```python
from build123d import *

# Parameters (mm, degrees)
CROQUIS1_W              = 30
CROQUIS1_H              = 30
SALIENTE_EXTRUIR1_DEPTH = 200
CROQUIS2_R              = 2
CORTAR_EXTRUIR1_DEPTH   = 25
CROQUIS3_R              = 2
CORTAR_EXTRUIR2_DEPTH   = 203.792997907
CROQUIS4_R              = 2
CORTAR_EXTRUIR3_DEPTH   = 25


with BuildPart() as part:
    # Croquis1 → Saliente-Extruir1 (new body)
    with BuildSketch(Plane.XY):
        Rectangle(CROQUIS1_W, CROQUIS1_H)
    extrude(amount=SALIENTE_EXTRUIR1_DEPTH)

    # Croquis2 → Cortar-Extruir1 (cut)
    with BuildSketch(Plane.XY.offset(200)):
        with Locations((-7.221825407, 7.221825407)):
            Circle(CROQUIS2_R)
        with Locations(Location((7.221825407, -7.221825407, 0), (0, 0, 180))):
            Circle(CROQUIS2_R)
    extrude(amount=-CORTAR_EXTRUIR1_DEPTH, mode=Mode.SUBTRACT)

    # Croquis3 → Cortar-Extruir2 (cut, through all)
    with BuildSketch(Plane(origin=(0, 15, 0), x_dir=(1, 0, 0), z_dir=(0, 1, 0))):
        with Locations(Location((0, -196, 0), (0, 0, 270))):
            Circle(CROQUIS3_R)
    extrude(amount=-CORTAR_EXTRUIR2_DEPTH, mode=Mode.SUBTRACT)

    # Croquis4 → Cortar-Extruir3 (cut)
    with BuildSketch(Plane(origin=(0, 0, 0), x_dir=(-1, 0, 0), z_dir=(0, 0, -1))):
        Circle(CROQUIS4_R)
    extrude(amount=-CORTAR_EXTRUIR3_DEPTH, mode=Mode.SUBTRACT)


solid = part.part
```
Input: part model. Units: mm. Frame: model coordinates. A direction names the side the tool comes from. Coordinates: 2 decimals unless noted, no trailing zeros. Loops run counter-clockwise (first coordinate to the right, second up) from the corner with the lowest first, then second, coordinate; pieces in that order, holes last. Notation, with made-up numbers: (-12, 71.25) -> (11, 71.25) arc R17 ccw to (11, 95.25) -> close; hole circle Ø10 at (85, -12.75). An arc over 180 degrees is marked (long way). Use a Markdown table: item, result.
1) Access query for faces 4 (the cylindrical face through (9.22, -7.31, 187.68)), 5 (the cylindrical face through (0, -2, 12)), 6 (the cylindrical face through (0, 0, 194)). Directions: +Z, -Z, +X, -X, +Y, -Y. A direction counts if a zero-diameter tool reaches every point of the face in a straight line with its end or side. Return the directions, or none.
Results found:
| item | result |
|---|---|
| face 4 | +Z |
| face 5 | -Z |
| face 6 | +Y, -Y |
2) Contact query for flat-ended pins moving along their axis: pin 1 (2.5 mm diameter, centred on x = 0, y = 0, fed in from -Z); pin 2 (3 mm diameter, centred on x = -7, y = 6.5, fed in from +Z). Output: stop coordinate, or through.
Results found:
| item | result |
|---|---|
| pin 1 | stops at z = 25 |
| pin 2 | stops at z = 200 |
3) Material intervals for line 1 along X through (y, z) = (-7, 196); line 2 along Y through (x, z) = (0, 13.75), sorted ascending. Write a range as from..to.
Results found:
| item | result |
|---|---|
| line 1 | x = -15..-2, 2..5.23, 9.21..15 |
| line 2 | y = -15..-2, 2..15 |
4) Cut plane B-B (z = 196). Return the cut outline in (x, y), then the cut area to 3 significant figures.
Results found:
| item | result |
|---|---|
| outline | (-15, -15) -> (-2, -15) -> (-2, 15) -> (-15, 15) -> close; (2, -15) -> (15, -15) -> (15, 15) -> (2, 15) -> close; hole circle Ø4 at (-7.22, 7.22); hole circle Ø4 at (7.22, -7.22) |
| area | 755 mm2 |
5) Pull-direction query (Y, two-part tool) for faces 1 (the flat face through (0, -15, 99)), 2 (the flat face through (-4, 0, 0)), 3 (the flat face through (0, 0, 25)); classes: released by +Y, released by -Y, zero draft, split by the parting line, or undercut.
Results found:
| item | result |
|---|---|
| face 1 | released by -Y |
| face 2 | zero draft |
| face 3 | undercut |
6) Cut plane A-A (x = 0). Return the cut outline in (y, z).
Results found:
| item | result |
|---|---|
| outline | (-15, 0) -> (-2, 0) -> (-2, 25) -> (2, 25) -> (2, 0) -> (15, 0) -> (15, 194) -> (-15, 194) -> close; (-15, 198) -> (15, 198) -> (15, 200) -> (-15, 200) -> close |
7) Cut plane C-C (y = 0). Return the cut outline in (x, z), then the cut area to 3 significant figures.
Results found:
| item | result |
|---|---|
| outline | (-15, 0) -> (-2, 0) -> (-2, 25) -> (2, 25) -> (2, 0) -> (15, 0) -> (15, 200) -> (-15, 200) -> close; hole circle Ø4 at (0, 196) |
| area | 5,890 mm2 |
